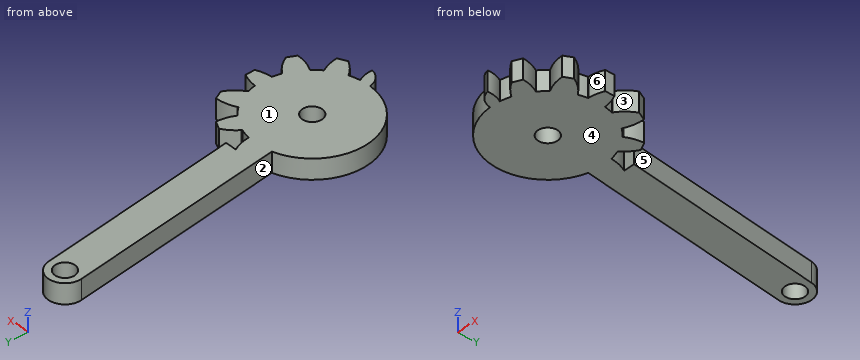
from build123d import *

# Parameters (mm, degrees)
SKETCH1_R           = 1.5
BOSS_EXTRUDE1_DEPTH = 3


with BuildPart() as part:
    # Sketch1 → Boss-Extrude1 (new body)
    with BuildSketch(Plane.XY.offset(1.9)):
        with BuildLine():
            Line((-6.319804534, 40.514327491), (-2.33662546, 8.172526015))
            ThreePointArc((-2.33662546, 8.172526015), (-8.436254395, -1.03904369), (-0.283752271, -8.495262483))
            ThreePointArc((-0.283752271, -8.495262483), (0.387258031, -9.932027081), (1.787569077, -10.676121371))
            ThreePointArc((1.787569077, -10.676121371), (1.706000613, -9.502192185), (1.28944453, -8.401626795))
            ThreePointArc((1.28944453, -8.401626795), (2.079332338, -8.241745994), (2.850528183, -8.007776788))
            ThreePointArc((2.850528183, -8.007776788), (3.779603703, -9.013165462), (4.91238571, -9.781795823))
            Line((4.91238571, -9.781795823), (6.178855756, -9.161994546))
            ThreePointArc((6.178855756, -9.161994546), (5.965894349, -7.885306169), (5.484085843, -6.683995909))
            Line((5.484085843, -6.683995909), (5.414116812, -6.552658937))
            ThreePointArc((5.414116812, -6.552658937), (6.01040764, -6.01040764), (6.552658937, -5.414116812))
            Line((6.552658937, -5.414116812), (6.683995909, -5.484085843))
            ThreePointArc((6.683995909, -5.484085843), (8.057590144, -6.011450066), (9.518230762, -6.188659346))
            Line((9.518230762, -6.188659346), (10.138032038, -4.922189299))
            ThreePointArc((10.138032038, -4.922189299), (9.323454041, -3.667986658), (8.224003874, -2.65419629))
            Line((8.224003874, -2.65419629), (8.102883181, -2.567739114))
            ThreePointArc((8.102883181, -2.567739114), (8.278718168, -1.926869349), (8.403949047, -1.274221493))
            Line((8.403949047, -1.274221493), (8.552369893, -1.263436399))
            ThreePointArc((8.552369893, -1.263436399), (9.641452494, -1.082458564), (10.678939324, -0.705))
            Line((10.678939324, -0.705), (10.678939324, 0.705))
            ThreePointArc((10.678939324, 0.705), (9.641452494, 1.082458564), (8.552369893, 1.263436399))
            Line((8.552369893, 1.263436399), (8.403949047, 1.274221493))
            ThreePointArc((8.403949047, 1.274221493), (8.278718168, 1.926869349), (8.102883181, 2.567739114))
            Line((8.102883181, 2.567739114), (8.224003874, 2.65419629))
            ThreePointArc((8.224003874, 2.65419629), (9.323454041, 3.667986658), (10.138032038, 4.922189299))
            Line((10.138032038, 4.922189299), (9.518230762, 6.188659346))
            ThreePointArc((9.518230762, 6.188659346), (8.057590144, 6.011450066), (6.683995909, 5.484085843))
            Line((6.683995909, 5.484085843), (6.552658937, 5.414116812))
            ThreePointArc((6.552658937, 5.414116812), (6.01040764, 6.01040764), (5.414116812, 6.552658937))
            Line((5.414116812, 6.552658937), (5.484085843, 6.683995909))
            ThreePointArc((5.484085843, 6.683995909), (5.965894349, 7.885306169), (6.178855756, 9.161994546))
            Line((6.178855756, 9.161994546), (4.91238571, 9.781795823))
            ThreePointArc((4.91238571, 9.781795823), (3.893417709, 9.032482418), (3.054167872, 8.08621286))
            Line((3.054167872, 8.08621286), (2.967710696, 7.965092167))
            ThreePointArc((2.967710696, 7.965092167), (2.199961883, 8.210369523), (1.41243323, 8.381827508))
            Line((1.41243323, 8.381827508), (1.401648136, 8.530248353))
            ThreePointArc((1.401648136, 8.530248353), (1.171954356, 9.79405056), (0.678518537, 10.980000113))
            Line((0.678518537, 10.980000113), (2.3553868, 10.980000113))
            Line((2.3553868, 10.980000113), (-1.357298788, 41.125503992))
            ThreePointArc((-1.357298788, 41.125503992), (-4.144139911, 43.301168615), (-6.319804534, 40.514327491))
        make_face()
        with Locations((-3.838551661, 40.819915742)):
            Circle(SKETCH1_R, mode=Mode.SUBTRACT)
        Circle(SKETCH1_R, mode=Mode.SUBTRACT)
    extrude(amount=-BOSS_EXTRUDE1_DEPTH)


solid = part.part
Geometry check sheet. Reference: the model listing, model coordinates, mm. Face numbers are marked on the shaded views. A direction names the side the tool comes from. Round coordinates to 2 decimals unless told otherwise and drop trailing zeros. Write each loop counter-clockwise with the first axis right and the second up, starting at its lowest first coordinate (ties: lowest second). Pieces come first, ordered by that corner, then holes.
Item 1: Mould release check, pull along Y, two halves, no side actions. Record for the marked faces 4, 5 and 6: +Y half, -Y half, draft (parallel to the pull), parting line (faces both ways), or undercut.
Determined:
face 4: draft
face 5: +Y half
face 6: undercut
Item 2: Section check A-A (y = 0). Record the boundary of the cut face in (x, z).
Determined:
outline: (-8.5, -1.1) - (-1.5, -1.1) - (-1.5, 1.9) - (-8.5, 1.9) - close; (1.5, -1.1) - (10.68, -1.1) - (10.68, 1.9) - (1.5, 1.9) - close
Item 3: Material ranges on line 1 along Y through (x, z) = (9.5, 1.65); line 2 along Y through (x, z) = (8.5, 1.75); line 3 along Y through (x, z) = (6.5, 0.95), recorded low to high.
Determined:
line 1: y = -6.19 to -3.89, -1.12 to 1.12, 3.89 to 6.19
line 2: y = -6.1 to -2.86, -1.27 to 1.27, 2.86 to 6.1
line 3: y = -5.48 to 5.48
Item 4: Access from +Z, -Z, +X, -X, +Y, -Y to the whole of each face (thin tool, end or side, straight path). Record for the marked faces 1, 2 and 3.
Determined:
face 1: +Z, +X, -X, +Y, -Y
face 2: +Z, -Z, -X
face 3: +Z, -Z, +X
Item 5: Section check B-B (z = 1.4). Give the number of separate pieces and of enclosed holes in the cut face, plus the area to 3 significant figures.
Determined:
separate pieces: 1
enclosed holes: 2
area: 417 mm2
Item 6: Go/stop test with flat-tipped pins: pin 1 Ø1.5 at (x, z) = (3.5, -0.5) entering from +Y; pin 2 Ø3.5 at (x, y) = (0, 0) entering from +Z. Record where each tip stops, or that it passes through.
Determined:
pin 1: stops at y = 9.33
pin 2: stops at z = 1.9
